The model under review builds one solid part; all positions refer to its coordinate system, in mm. Face numbers are marked on the shaded views. A direction names the side the tool comes from. Give positions to 0.01 mm unless a question says otherwise; leave off trailing zeros. Write each loop counter-clockwise with the first axis right and the second up, starting at its lowest first coordinate (ties: lowest second). Pieces come first, ordered by that corner, then holes. Notation, with made-up numbers: (-37.5, 69) - (1.5, 69) arc R20 cw to (1.5, 84) - close; hole circle Ø1 at (-5.75, 27.5). An arc over 180 degrees is marked (long way). Write item = value, one per line.
```python
from build123d import *

# Parameters (mm, degrees)
F1_DEPTH  = 203.2
F2_W      = 25.4
F2_H      = 25.4
F3_DEPTH  = 177.8
F5_DEPTH  = 152.4
F7_DEPTH  = 127
F9_DEPTH  = 101.6
F11_DEPTH = 76.2
F13_DEPTH = 50.8
F15_DEPTH = 25.4
F16_R     = 0.508
F17_DEPTH = 190.5
F18_R     = 0.381
F19_DEPTH = 215.9
F20_R     = 0.635
F21_DEPTH = 165.1


with BuildPart() as f1:
    # F0 (on Front) → F1 (new body)
    with BuildSketch(Plane.XZ):
        Polygon((-12.7, -7.332348), (12.7, -7.332348), (0, 14.664697), align=None)
    extrude(amount=F1_DEPTH)

    # F2 (on Front) → F3 (join)
    with BuildSketch(Plane.XZ):
        with Locations((0, 5.367652)):
            Rectangle(F2_W, F2_H)
    extrude(amount=F3_DEPTH)

    # F4 (on Front) → F5 (join)
    with BuildSketch(Plane.XZ):
        Polygon((-12.7, -7.332348), (12.7, -7.332348), (20.549032, 16.824487), (0, 31.754233), (-20.549032, 16.824487), align=None)
    extrude(amount=F5_DEPTH)

    # F6 (on Front) → F7 (join)
    with BuildSketch(Plane.XZ):
        Polygon((-12.7, -7.332348), (12.7, -7.332348), (25.4, 14.664697), (12.7, 36.661742), (-12.7, 36.661742), (-25.4, 14.664697), align=None)
    extrude(amount=F7_DEPTH)

    # F8 (on Front) → F9 (join)
    with BuildSketch(Plane.XZ):
        Polygon((-12.7, -7.332348), (12.7, -7.332348), (28.536641, 12.526171), (22.884609, 37.28934), (0, 48.309987), (-22.884609, 37.28934), (-28.536641, 12.526171), align=None)
    extrude(amount=F9_DEPTH)

    # F10 (on Front) → F11 (join)
    with BuildSketch(Plane.XZ):
        Polygon((-12.7, -7.332348), (12.7, -7.332348), (30.660512, 10.628164), (30.660512, 36.028164), (12.7, 53.988676), (-12.7, 53.988676), (-30.660512, 36.028164), (-30.660512, 10.628164), align=None)
    extrude(amount=F11_DEPTH)

    # F12 (on Front) → F13 (join)
    with BuildSketch(Plane.XZ):
        Polygon((-12.7, -7.332348), (12.7, -7.332348), (32.157529, 8.994457), (36.568193, 34.008574), (23.868193, 56.005619), (0, 64.692931), (-23.868193, 56.005619), (-36.568193, 34.008574), (-32.157529, 8.994457), align=None)
    extrude(amount=F13_DEPTH)

    # F14 (on Front) → F15 (join)
    with BuildSketch(Plane.XZ):
        Polygon((-12.7, -7.332348), (12.7, -7.332348), (33.249032, 7.597397), (41.098063, 31.754233), (33.249032, 55.911068), (12.7, 70.840813), (-12.7, 70.840813), (-33.249032, 55.911068), (-41.098063, 31.754233), (-33.249032, 7.597397), align=None)
    extrude(amount=F15_DEPTH)

    # F16 (on face) → F17 (join)
    with BuildSketch(Plane.XZ.offset(177.8)):
        with Locations((0, 5.367652)):
            Circle(F16_R)
    extrude(amount=-F17_DEPTH)

    # F18 (on face) → F19 (join)
    with BuildSketch(Plane.XZ.offset(203.2)):
        Circle(F18_R)
    extrude(amount=-F19_DEPTH)

    # F20 (on face) → F21 (join)
    with BuildSketch(Plane.XZ.offset(152.4)):
        with Locations((0, 10.147702)):
            Circle(F20_R)
    extrude(amount=-F21_DEPTH)


solid = f1.part
```
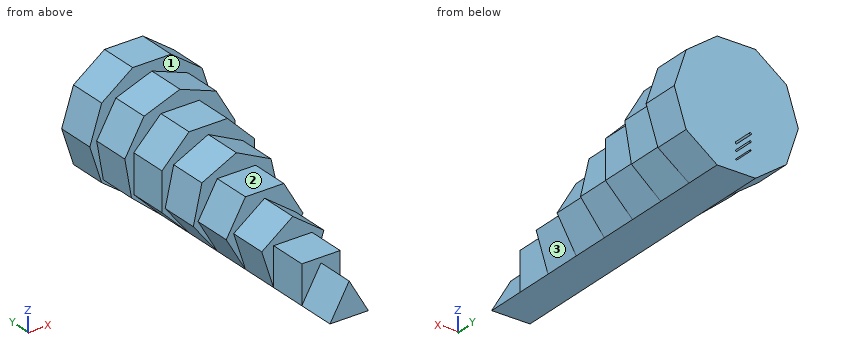
1. Take a section at A-A on y = -39.5. Give the boundary of the cut face in (x, z), and give its area (3 significant figures).
Findings below:
outline = (-36.57, 34.01) - (-32.16, 8.99) - (-12.7, -7.33) - (12.7, -7.33) - (32.16, 8.99) - (36.57, 34.01) - (23.87, 56.01) - (0, 64.69) - (-23.87, 56.01) - close
area = 3,990 mm²
2. Insertion check: P1, Ø12.5, axis at x = -5.5, y = -67.5, coming from the +Z side; P2, Ø2, axis at y = -80.5, z = 39.5, coming from the +X side; P3, Ø20.5, axis at x = -5, y = -111.5, coming from the +Z side; P4, Ø6, axis at y = -155.5, z = 31, coming from the -X side. Each pin has a flat end and moves straight along its axis. Give the tip position at first contact, or say it passes through.
Findings below:
P1 = 53.99
P2 = 20.37
P3 = 47.18
P4 = through
3. For line 1 (Y direction, x = 14, z = 40); line 2 (Y direction, x = -8.5, z = 66); line 3 (Z direction, x = -6, y = -171), list the stretches that pass through material, from the lowest coordinate up. Write a range as from..to.
Findings below:
line_1 = -101.6..0
line_2 = -25.4..0
line_3 = -7.33..18.07
4. Machinability: for the marked faces 1, 2 and 3, which of the approach directions +Z, -Z, +X, -X, +Y, -Y give a long, thin tool a straight path to every point of the face, cutting with its end or side? Answer none if there is none.
Findings below:
face_1 = -Y
face_2 = +Z, +X, -X, -Y
face_3 = -Z, +X, -Y
5. Take a section at C-C on y = -71. Give the boundary of the cut face in (x, z).
Findings below:
outline = (-30.66, 10.63) - (-12.7, -7.33) - (12.7, -7.33) - (30.66, 10.63) - (30.66, 36.03) - (12.7, 53.99) - (-12.7, 53.99) - (-30.66, 36.03) - close
6. Take a section at B-B on x = -17. Give the boundary of the cut face in (y, z), and give its area (3 significant figures).
Findings below:
outline = (-152.4, 5.9) - (-127, 5.9) - (-127, 0.12) - (-101.6, 0.12) - (-101.6, -1.94) - (-76.2, -1.94) - (-76.2, -3.03) - (-50.8, -3.03) - (-50.8, -3.72) - (-25.4, -3.72) - (-25.4, -4.21) - (0, -4.21) - (0, 67.72) - (-25.4, 67.72) - (-25.4, 58.51) - (-50.8, 58.51) - (-50.8, 49.69) - (-76.2, 49.69) - (-76.2, 40.12) - (-101.6, 40.12) - (-101.6, 29.21) - (-127, 29.21) - (-127, 19.4) - (-152.4, 19.4) - close
area = 6,900 mm²
